Geometry check sheet. Reference: drawing and pictorial views, mm from the part's lowest x, y, z. A direction names the side the tool comes from. Round coordinates to 2 decimals unless told otherwise and drop trailing zeros. Write each loop counter-clockwise with the first axis right and the second up, starting at its lowest first coordinate (ties: lowest second). Pieces come first, ordered by that corner, then holes. Notation, with made-up numbers: (85.25, 24.5) -> (114.25, 24.5) arc R18 ccw to (114.25, 48.5) -> close; hole circle Ø11 at (47.5, 5.25). An arc over 180 degrees is marked (long way). Write item = value, one per line.
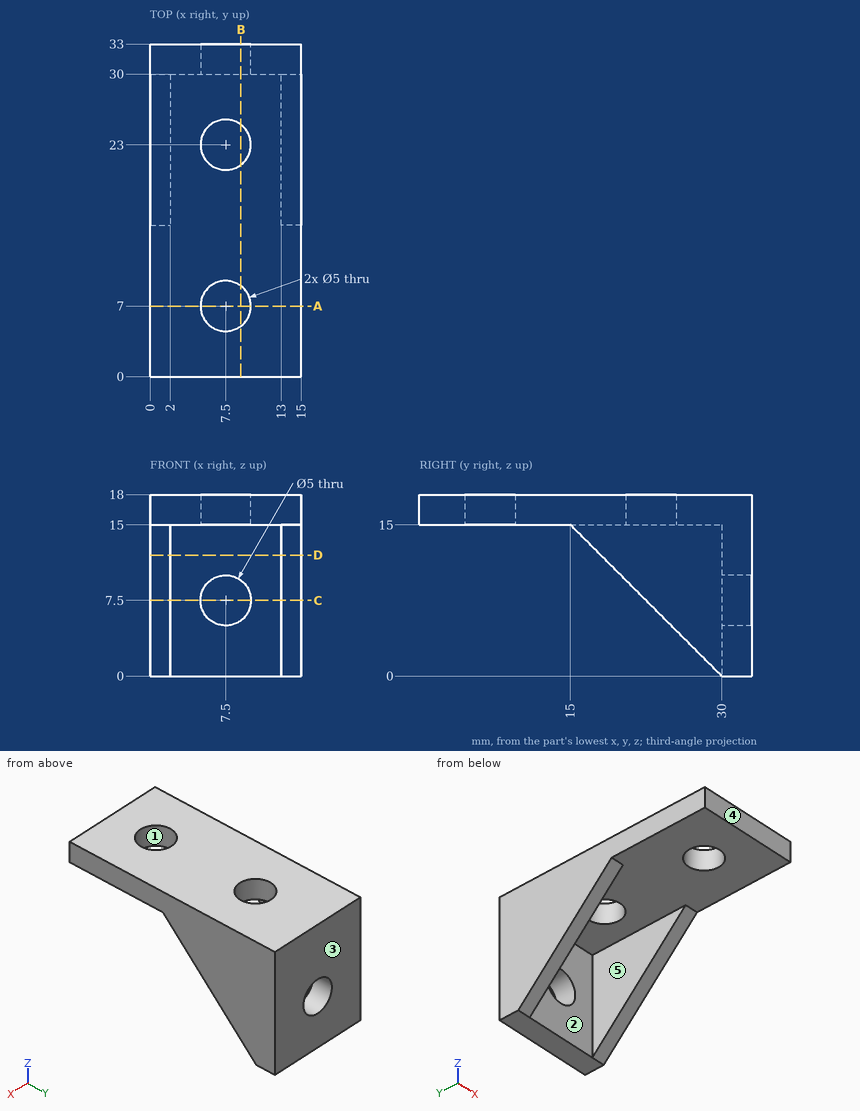
(1) Material ranges on L1, parallel to Y at x = 7.5, z = 16.15; L2, parallel to X at y = 21.5, z = 10.75; L3, parallel to X at y = 31.35, z = 7.5, recorded low to high. Write a range as [from, to].
Worked answers:
L1 = [0, 4.5], [9.5, 20.5], [25.5, 33]
L2 = [0, 2], [13, 15]
L3 = [0, 5], [10, 15]
(2) Sectioned sample at A-A on y = 7. Enter the section's corners in (x, z).
Worked answers:
outline = (0, 15) -> (5, 15) -> (5, 18) -> (0, 18) -> close; (10, 15) -> (15, 15) -> (15, 18) -> (10, 18) -> close
(3) Go/stop test with flat-tipped pins: P1, Ø4, axis at x = 2.5, y = 19.5, coming from the -Z side; P2, Ø5, axis at x = 2, y = 20, coming from the -Z side; P3, Ø1.5, axis at x = 13, z = 7.5, coming from the -Y side. Record where each tip stops, or that it passes through.
Worked answers:
P1 = 8.56
P2 = 7.5
P3 = 21.75
(4) Sectioned sample at D-D on z = 12. Enter the section's corners in (x, y), then the cut area to 3 significant figures.
Worked answers:
outline = (0, 18) -> (2, 18) -> (2, 30) -> (13, 30) -> (13, 18) -> (15, 18) -> (15, 33) -> (0, 33) -> close
area = 93.0 mm²
(5) Access from +Z, -Z, +X, -X, +Y, -Y to the whole of each face (thin tool, end or side, straight path). Record for the marked faces 4 and 5.
Worked answers:
face_4 = +Z, -Z, +X, -X, -Y
face_5 = -Z, -Y
(6) Release check for a two-part mould opening along Y. For the marked faces 1, 2 and 3 record: pulls with the +Y half, pulls with the -Y half, needs draft (parallel to the pull), parting line crosses it, or undercut.
Worked answers:
face_1 = undercut
face_2 = pulls with the -Y half
face_3 = pulls with the +Y half
(7) Sectioned sample at B-B on x = 9. Enter the section's corners in (y, z), then the cut area to 3 significant figures.
Worked answers:
outline = (0, 15) -> (5, 15) -> (5, 18) -> (0, 18) -> close; (9, 15) -> (21, 15) -> (21, 18) -> (9, 18) -> close; (25, 15) -> (30, 15) -> (30, 9.5) -> (33, 9.5) -> (33, 18) -> (25, 18) -> close; (30, 0) -> (33, 0) -> (33, 5.5) -> (30, 5.5) -> close
area = 108 mm²
(8) Sectioned sample at C-C on z = 7.5. Enter the section's corners in (x, y).
Worked answers:
outline = (0, 22.5) -> (2, 22.5) -> (2, 30) -> (5, 30) -> (5, 33) -> (0, 33) -> close; (10, 30) -> (13, 30) -> (13, 22.5) -> (15, 22.5) -> (15, 33) -> (10, 33) -> close
